Model file for the job. Use its own axes, mm. A direction names the side the tool comes from. Give positions to 0.01 mm unless a question says otherwise; leave off trailing zeros. Write each loop counter-clockwise with the first axis right and the second up, starting at its lowest first coordinate (ties: lowest second). Pieces come first, ordered by that corner, then holes. Notation, with made-up numbers: (-24.5, 41.25) - (7.5, 41.25) arc R14 cw to (7.5, 45.25) - close; hole circle Ø3 at (-26.5, -11.5). An arc over 180 degrees is marked (long way). Use CSV: the item, a comma, the result in double quotes.
from build123d import *

# Parameters (mm, degrees)
SKETCH1_R           = 1.5
BOSS_EXTRUDE1_DEPTH = 3


with BuildPart() as part:
    # Sketch1 → Boss-Extrude1 (new body)
    with BuildSketch(Plane.XY):
        with BuildLine():
            ThreePointArc((-32.534155724, 4.476054283), (-33.095330262, 0.22593084), (-32.534155724, -4.024192603))
            ThreePointArc((-32.534155724, -4.024192603), (-16.720330262, -13.19906916), (-0.906504801, -4.024192603))
            ThreePointArc((-0.906504801, -4.024192603), (-0.345330262, 0.22593084), (-0.906504801, 4.476054283))
            ThreePointArc((-0.906504801, 4.476054283), (-16.720330262, 13.65093084), (-32.534155724, 4.476054283))
        make_face()
        with Locations((-2.845330262, 0.22593084)):
            Circle(SKETCH1_R, mode=Mode.SUBTRACT)
        with Locations((-30.595330262, 0.22593084)):
            Circle(SKETCH1_R, mode=Mode.SUBTRACT)
        with BuildLine():
            Line((-28.010508516, -1.52406916), (-25.930548772, -1.52406916))
            ThreePointArc((-25.930548772, -1.52406916), (-26.095330262, 0.22593084), (-25.930548772, 1.97593084))
            Line((-25.930548772, 1.97593084), (-28.010508516, 1.97593084))
            ThreePointArc((-28.010508516, 1.97593084), (-16.720330262, 11.65093084), (-5.430152009, 1.97593084))
            Line((-5.430152009, 1.97593084), (-7.510111752, 1.97593084))
            ThreePointArc((-7.510111752, 1.97593084), (-7.345330262, 0.22593084), (-7.510111752, -1.52406916))
            Line((-7.510111752, -1.52406916), (-5.430152009, -1.52406916))
            ThreePointArc((-5.430152009, -1.52406916), (-16.720330262, -11.19906916), (-28.010508516, -1.52406916))
        make_face(mode=Mode.SUBTRACT)
    extrude(amount=BOSS_EXTRUDE1_DEPTH)


solid = part.part
(1) Wall check: probe 1 along X at (y, z) = (-0.25, 1.7); probe 2 along X at (y, z) = (1, 0.7); probe 3 along X at (y, z) = (-6.75, 1.4). Give the ranges that are in metal, low to high. Write a range as [from, to].
Checked values:
probe 1,"x = [-33.09, -32.02], [-29.17, -26.08], [-7.36, -4.27], [-1.42, -0.35]"
probe 2,"x = [-33.08, -31.88], [-29.31, -26.06], [-7.38, -4.13], [-1.56, -0.36]"
probe 3,"x = [-30.63, -25.77], [-7.67, -2.81]"
(2) Flat gauge pins, fed straight in: P1, Ø1.8, axis at x = -30.6, y = 0.23, coming from the -Z side (3 decimals); P2, Ø1, axis at x = -20.5, z = 0.5, coming from the -Y side; P3, Ø1.7, axis at x = -6.5, z = 1.5, coming from the -Y side; P4, Ø1.7, axis at x = -27, z = 2, coming from the +Y side. Where does each tip first touch, or does it go through?
Checked values:
P1,"passes through"
P2,"stops at y = -12.9"
P3,"stops at y = -10.6"
P4,"stops at y = 11.02"
(3) 3-axis set-ups, long thin cutter, end or side, ignore diameter. For faces 1 (the face through (-0.345, 0.166, 1.479)), 2 (the face through (-26.095, 0.201, 1.479)): which of +Z, -Z, +X, -X, +Y, -Y reach the whole face in a straight line?
Checked values:
face 1,"+Z, -Z, +X"
face 2,"+Z, -Z"
(4) Pull direction X, two halves, no side cores. Call faces 3 (the face through (-16.45, 13.65, 1.48)), 4 (the face through (-16.494, -11.197, 1.479)), 5 (the face through (-33.095, 0.286, 1.479)), 6 (the face through (-16.95, 11.65, 1.48)): released by +X, released by -X, zero draft, split by the parting line, or undercut.
Checked values:
face 3,"split by the parting line"
face 4,"undercut"
face 5,"released by -X"
face 6,"undercut"
(5) Saw through at A-A, the plane y = -9. List the corners of the cut face in (x, z), then the cut area to 3 significant figures.
Checked values:
outline,"(-28.35, 0) - (-23.46, 0) - (-23.46, 3) - (-28.35, 3) - close; (-9.98, 0) - (-5.09, 0) - (-5.09, 3) - (-9.98, 3) - close"
area,"29.4 mm^2"
(6) Saw through at C-C, the plane z = 1.2. Count the separate pieces of the cut face and the enclosed holes in it, then the cut area to 3 significant figures.
Checked values:
separate pieces,"1"
enclosed holes,"3"
area,"277 mm^2"
(7) Saw through at B-B, the plane x = -8. List the corners of the cut face in (y, z), then the cut area to 3 significant figures.
Checked values:
outline,"(-10.98, 0) - (-7.16, 0) - (-7.16, 3) - (-10.98, 3) - close; (7.61, 0) - (11.43, 0) - (11.43, 3) - (7.61, 3) - close"
area,"22.9 mm^2"
